Here's how the part is built. I have some questions about the finished solid (model axes, mm). A direction names the side the tool comes from. Round coordinates to 2 decimals unless told otherwise and drop trailing zeros. Loops run counter-clockwise (first coordinate to the right, second up) from the corner with the lowest first, then second, coordinate; pieces in that order, holes last. Notation, with made-up numbers: (11.25, 70) -> (59.25, 70) arc R27 ccw to (59.25, 106) -> close; hole circle Ø5 at (50.5, -39.5). An arc over 180 degrees is marked (long way). Use one line per item in the form item = value. Start each with the question number.
Item 1: If we section it at C-C (y = -35.5): Write out the boundary of the cut face in (x, z), then the cut area to 3 significant figures.
Item 2: If we section it at A-A (x = 0): Write out the boundary of the cut face in (y, z).
Item 3: If we section it at D-D (z = 110): Write out the boundary of the cut face in (x, y), then the cut area to 3 significant figures.
Item 4: If I drill on L1, parallel to Z at x = 0, y = -20; L2, parallel to Y at x = 128, z = 56.5; L3, parallel to Z at x = -110, y = 17, over which ranges is the centre line in solid material (lowest first)? Write a range as [from, to].
Item 5: If we section it at B-B (z = 45): Write out the boundary of the cut face in (x, y), then the cut area to 3 significant figures.
Item 6: For faces 1 (the face through (140, -1, 75)), 2 (the face through (144, -40, 57)), 3 (the face through (110, -40, -1)), which set-ups out of +Z, -Z, +X, -X, +Y, -Y let a thin tool reach every point of the face, with its end or its side?
Item 7: Thinking about a two-plate mould opening in X: for faces 4 (the face through (100, 1, 1)), 5 (the face through (150, -1, 1)), 6 (the face through (-112, 50, 56)), which applies, released by +X, released by -X, zero draft, split by the parting line, or undercut?
Item 8: I'm going to push flat-ended pins straight in: pin 1 Ø6 at (x, y) = (142, 10.5) entering from -Z; pin 2 Ø12 at (x, y) = (-83.5, 20) entering from -Z; pin 3 Ø5 at (y, z) = (-15.5, -107) entering from -X. Where does each tip first touch, or does it pass through?
```python
from build123d import *

# Parameters (mm, degrees)
F0_R     = 150
F1_DEPTH = 50
F2_R     = 125
F3_DEPTH = 100
F4_W     = 80
F4_H     = 150
F5_DEPTH = 150
F6_W     = 80
F6_H     = 150
F7_DEPTH = 100
F8_R     = 6.051989
F9_DEPTH = 10


with BuildPart() as f1:
    # F0 (on Front) → F1 (new body, symmetric)
    with BuildSketch(Plane.XZ):
        Circle(F0_R)
    extrude(amount=F1_DEPTH, both=True)

    # F2 (on face) → F3 (cut, through all)
    with BuildSketch(Plane.XZ.offset(50)):
        Circle(F2_R)
    extrude(amount=-F3_DEPTH, mode=Mode.SUBTRACT)

    # F4 (on Right) → F5 (join)
    with BuildSketch(Plane.YZ):
        Rectangle(F4_W, F4_H)
    extrude(amount=F5_DEPTH)

    # F6 (on face) → F7 (cut)
    with BuildSketch(Plane(origin=(0, 0, 0), x_dir=(0, -1, 0), z_dir=(-1, 0, 0))):
        Rectangle(F6_W, F6_H)
    extrude(amount=-F7_DEPTH, mode=Mode.SUBTRACT)

    # F8 (on face) → F9 (join)
    with BuildSketch(Plane(origin=(0, 50, 0), x_dir=(-1, 0, 0), z_dir=(0, 1, 0))):
        with Locations((-136, 0)):
            Circle(F8_R)
    extrude(amount=F9_DEPTH)


solid = f1.part
```
Values found:
q1.outline = (129.9, -75) -> (150, -75) -> (150, 75) -> (129.9, 75) arc R150 ccw (long way) to start; hole (100, -75) -> (100, 75) arc R125 ccw (long way) to start
q1.area = 25,100 mm2
q2.outline = (-50, -150) -> (50, -150) -> (50, -125) -> (-50, -125) -> close; (-50, 125) -> (50, 125) -> (50, 150) -> (-50, 150) -> close
q3.outline = (-101.98, -50) -> (-59.37, -50) -> (-59.37, 50) -> (-101.98, 50) -> close; (59.37, -50) -> (101.98, -50) -> (101.98, 50) -> (59.37, 50) -> close
q3.area = 8,520 mm2
q4.L1 = [-150, -125], [125, 150]
q4.L2 = [-50, 50]
q4.L3 = [-101.98, -59.37], [59.37, 101.98]
q5.outline = (-143.09, -50) -> (-116.62, -50) -> (-116.62, 50) -> (-143.09, 50) -> close; (100, -40) -> (116.62, -40) -> (116.62, -50) -> (143.09, -50) -> (143.09, -40) -> (150, -40) -> (150, 40) -> (143.09, 40) -> (143.09, 50) -> (116.62, 50) -> (116.62, 40) -> (100, 40) -> close
q5.area = 7,180 mm2
q6.face_1 = +Z, +X, +Y, -Y
q6.face_2 = +Z, +X, -Y
q6.face_3 = -Y
q7.face_4 = undercut
q7.face_5 = released by +X
q7.face_6 = zero draft
q8.pin_1 = -75
q8.pin_2 = -128.43
q8.pin_3 = -107.61
